```python
from build123d import *

# Parameters (mm, degrees)
F0_W      = 250
F0_H      = 250
F0_W_2    = 200
F0_H_2    = 200
F1_DEPTH  = 125
F2_W      = 200
F2_H      = 200
F3_DEPTH  = 100
F4_W      = 200
F4_H      = 200
F5_DEPTH  = 20
F6_W      = 200
F6_H      = 200
F7_DEPTH  = 20
F8_W      = 200
F8_H      = 200
F9_DEPTH  = 20
F10_W     = 200
F10_H     = 200
F11_DEPTH = 20
F12_R     = 1
F13_W     = 23
F13_H     = 23
F14_DEPTH = 4
F15_W     = 23
F15_H     = 23
F16_DEPTH = 4
F17_W     = 23
F17_H     = 23
F18_DEPTH = 4


with BuildPart() as f1:
    # F0 (on Front) → F1 (new body, symmetric)
    with BuildSketch(Plane.XZ):
        with Locations((125, 125)):
            Rectangle(F0_W, F0_H)
        with Locations((125, 125)):
            Rectangle(F0_W_2, F0_H_2, mode=Mode.SUBTRACT)
    extrude(amount=F1_DEPTH, both=True)

    # F2 (on Front) → F3 (join, symmetric)
    with BuildSketch(Plane.XZ):
        with Locations((125, 125)):
            Rectangle(F2_W, F2_H)
    extrude(amount=F3_DEPTH, both=True)

    # F4 (on face) → F5 (cut)
    with BuildSketch(Plane(origin=(0, 0, 0), x_dir=(0, -1, 0), z_dir=(-1, 0, 0))):
        with Locations((0, 125)):
            Rectangle(F4_W, F4_H)
    extrude(amount=-F5_DEPTH, mode=Mode.SUBTRACT)

    # F6 (on face) → F7 (cut)
    with BuildSketch(Plane.YZ.offset(250)):
        with Locations((0, 125)):
            Rectangle(F6_W, F6_H)
    extrude(amount=-F7_DEPTH, mode=Mode.SUBTRACT)

    # F8 (on Top) → F9 (cut)
    with BuildSketch(Plane.XY):
        with Locations((125, 0)):
            Rectangle(F8_W, F8_H)
    extrude(amount=F9_DEPTH, mode=Mode.SUBTRACT)

    # F10 (on face) → F11 (cut)
    with BuildSketch(Plane.XY.offset(250)):
        with Locations((125, 0)):
            Rectangle(F10_W, F10_H)
    extrude(amount=-F11_DEPTH, mode=Mode.SUBTRACT)

    # F12
    f12_edges = [f1.edges().sort_by_distance(p)[0] for p in [
        (25, 0, 0),
        (125, -100, 0),
        (125, 100, 0),
        (225, 0, 0),
        (250, 0, 0),
        (250, 0, 25),
        (250, 100, 125),
        (250, 0, 225),
        (250, -100, 125),
        (250, -125, 125),
        (250, 0, 250),
        (125, 125, 250),
        (250, 125, 125),
        (225, 125, 125),
        (125, 125, 225),
        (25, 125, 125),
        (125, 125, 25),
        (0, 100, 125),
        (0, 0, 25),
        (0, 125, 125),
        (0, 0, 0),
        (0, -125, 125),
        (0, 0, 250),
        (0, 0, 225),
        (0, -100, 125),
        (125, -125, 250),
        (125, -125, 0),
        (25, -125, 125),
        (125, -125, 225),
        (225, -125, 125),
        (125, -125, 25),
        (125, 100, 250),
        (25, 0, 250),
        (125, -100, 250),
        (225, 0, 250),
    ]]
    fillet(f12_edges, radius=F12_R)

    # F13 (on face) → F14 (join)
    with BuildSketch(Plane.XY.offset(250)):
        with Locations((237.5, 112.5)):
            Rectangle(F13_W, F13_H)
        with Locations((237.5, -112.5)):
            Rectangle(F13_W, F13_H)
        with Locations((12.5, -112.5)):
            Rectangle(F13_W, F13_H)
        with Locations((12.5, 112.5)):
            Rectangle(F13_W, F13_H)
    extrude(amount=F14_DEPTH)

    # F15 (on face) → F16 (join)
    with BuildSketch(Plane.YZ.offset(250)):
        Polygon((124, 224), (124, 249), (101, 249), (101, 226), (101, 224), align=None)
        Polygon((-101, 226), (-101, 249), (-124, 249), (-124, 224), (-101, 224), align=None)
        with Locations((-112.5, 12.5)):
            Rectangle(F15_W, F15_H)
        with Locations((112.5, 12.5)):
            Rectangle(F15_W, F15_H)
    extrude(amount=F16_DEPTH)

    # F17 (on face) → F18 (join)
    with BuildSketch(Plane(origin=(0, 125, 0), x_dir=(-1, 0, 0), z_dir=(0, 1, 0))):
        with Locations((-12.5, 12.5)):
            Rectangle(F17_W, F17_H)
        Polygon((-224, 1), (-224, 24), (-226, 24), (-249, 24), (-249, 1), align=None)
        Polygon((-224, 226), (-224, 249), (-249, 249), (-249, 226), (-226, 226), align=None)
        with Locations((-12.5, 237.5)):
            Rectangle(F17_W, F17_H)
    extrude(amount=F18_DEPTH)


solid = f1.part
```
CAD build for the part. Positions are in the model's coordinates, mm. A direction names the side the tool comes from. Round coordinates to 2 decimals unless told otherwise and drop trailing zeros. Use a Markdown table: item, result. Add a question column.
(1) Which spindle directions (+Z, -Z, +X, -X, +Y, -Y) get a long thin tool onto all of the face, cutting with end or side? Do faces 4 (the face through (124, 100, 240)), 5 (the face through (124, 112, 250)), 6 (the face through (124, -112, 225)), 7 (the face through (250, -1, 12)), 8 (the face through (240, -1, 25)). Say none if no direction does.
(2) Drill centre lines: line 1 (Y direction, x = 17, z = 158.5); line 2 (Z direction, x = 82, y = -101.5); line 3 (Z direction, x = 70.5, y = 60.5). Where is each one in solid material? Low to high.
(3) Pull direction X, two halves, no side cores. Call faces 1 (the face through (250, 112, 123)), 2 (the face through (225, -112, 124)), 3 (the face through (237, -1, 250)): +X half, -X half, draft (parallel to the pull), parting line (faces both ways), or undercut.
(4) Flat gauge pins, fed straight in: pin 1 (3 mm diameter, centred on x = 252.5, z = 17, fed in from +Y); pin 2 (8 mm diameter, centred on x = 197, y = -29, fed in from -Z); pin 3 (1.5 mm diameter, centred on x = 108.5, z = 105, fed in from +Y). Where does each tip first touch, or does it go through?
Geometry says:
| question | item | result |
|---|---|---|
| 1 | face 4 | +Z |
| 1 | face 5 | +Z, +Y, -Y |
| 1 | face 6 | -Y |
| 1 | face 7 | +Z, -Z, +X |
| 1 | face 8 | +X |
| 2 | line 1 | y = -125 to -100, 100 to 125 |
| 2 | line 2 | z = 0 to 25, 225 to 250 |
| 2 | line 3 | z = 20 to 230 |
| 3 | face 1 | +X half |
| 3 | face 2 | undercut |
| 3 | face 3 | draft |
| 4 | pin 1 | stops at y = 124 |
| 4 | pin 2 | stops at z = 20 |
| 4 | pin 3 | stops at y = 100 |
